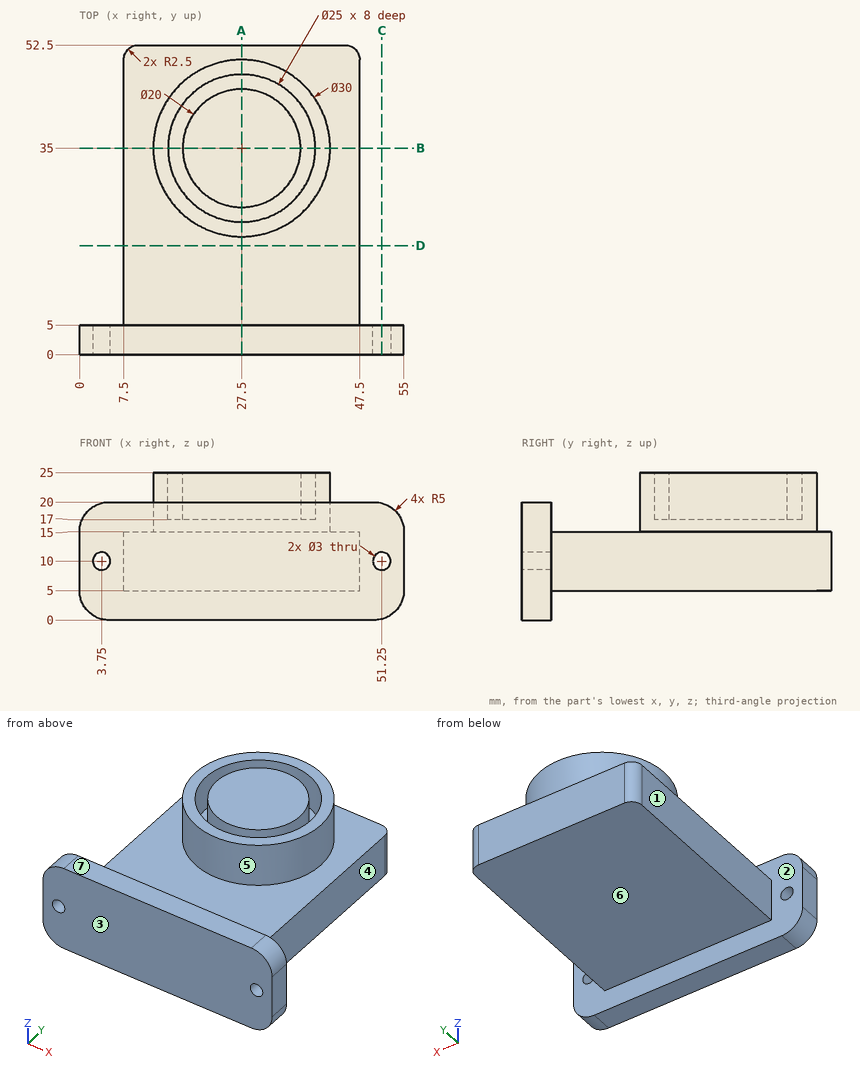
Job drawing, mm, ordinate dimensions from the low corner. One solid piece. A direction names the side the tool comes from. Round coordinates to 2 decimals unless told otherwise and drop trailing zeros. Loops run counter-clockwise (first coordinate to the right, second up) from the corner with the lowest first, then second, coordinate; pieces in that order, holes last.
Item 1: 3-axis set-ups, long thin cutter, end or side, ignore diameter. For the marked faces 4, 5, 6 and 7: which of +Z, -Z, +X, -X, +Y, -Y reach the whole face in a straight line?
Item 2: Cut at D-D, the plane y = 18.5. Give the cut face in (x, z), then the cut area to 3 significant figures.
Item 3: Cut at C-C, the plane x = 51.25. Give the cut face in (y, z).
Item 4: Drill centre lines: line 1 (Y direction, x = 27.5, z = 22.5); line 2 (Z direction, x = 40, y = 47); line 3 (X direction, y = 15, z = 7.5). Where is each one in solid material? Low to high.
Item 5: Mould opens along Y. For the marked faces 1, 2 and 3 say: +Y half, -Y half, draft (parallel to the pull), parting line (faces both ways), or undercut.
Item 6: Cut at A-A, the plane x = 27.5. Give the cut face in (y, z).
Item 7: Drop flat-ended pins along their axis: P1, Ø5, axis at y = 37, z = 12, coming from the +X side; P2, Ø8, axis at x = 34.5, y = 22, coming from the -Z side; P3, Ø1, axis at x = 9.5, z = 6.5, coming from the -Y side; P4, Ø5.5, axis at x = 18.5, y = 1.5, coming from the +Z side. Give the stop position or say it passes through.
Item 8: Cut at B-B, the plane y = 35. Give the cut face in (x, z), then the cut area to 3 significant figures.
A:
1. face 4: +Z, -Z, +X, +Y
1. face 5: +Z
1. face 6: -Z, +X, -X, +Y
1. face 7: +Z, +X, -X, -Y
2. outline: (7.5, 5) - (47.5, 5) - (47.5, 15) - (7.5, 15) - close
2. area: 400 mm2
3. outline: (0, 0.16) - (5, 0.16) - (5, 8.5) - (0, 8.5) - close; (0, 11.5) - (5, 11.5) - (5, 19.84) - (0, 19.84) - close
4. line 1: y = 20 to 22.5, 25 to 45, 47.5 to 50
4. line 2: z = 5 to 15
4. line 3: x = 7.5 to 47.5
5. face 1: draft
5. face 2: undercut
5. face 3: -Y half
6. outline: (0, 0) - (5, 0) - (5, 5) - (52.5, 5) - (52.5, 15) - (50, 15) - (50, 25) - (47.5, 25) - (47.5, 17) - (45, 17) - (45, 25) - (25, 25) - (25, 17) - (22.5, 17) - (22.5, 25) - (20, 25) - (20, 15) - (5, 15) - (5, 20) - (0, 20) - close
7. P1: stops at x = 47.5
7. P2: stops at z = 5
7. P3: stops at y = 0
7. P4: stops at z = 20
8. outline: (7.5, 5) - (47.5, 5) - (47.5, 15) - (42.5, 15) - (42.5, 25) - (40, 25) - (40, 17) - (37.5, 17) - (37.5, 25) - (17.5, 25) - (17.5, 17) - (15, 17) - (15, 25) - (12.5, 25) - (12.5, 15) - (7.5, 15) - close
8. area: 660 mm2
